```python
from build123d import *

# Parameters (mm, degrees)
SKETCH1_W            = 42
SKETCH1_H            = 33.02
BOSS_EXTRUDE1_DEPTH  = 0.381
SKETCH3_R            = 1.2192
CUT_EXTRUDE2_DEPTH   = 1.5875
CUT_EXTRUDE1_REACH   = 28.724
CUT_EXTRUDE3_START   = -0.762
CUT_EXTRUDE3_DEPTH   = 0.762
FILLET1_R            = 1.27
CUT_EXTRUDE4_REACH   = 28.724
SKETCH7_R            = 0.7874
FILLET1_OF_MIRROR1_R = 1.27
MIRROR2_START        = -0.381
MIRROR2_DEPTH        = 0.762
SKETCH6_W            = 2.5
SKETCH6_H            = 9.525
BOSS_EXTRUDE2_DEPTH  = 0.0254
CIRPATTERN1_COUNT    = 2


# Read off the part's stored shape, not the designer's step: Mirror2
with BuildPart() as part:
    # Sketch1 → Boss-Extrude1 (new, symmetric)
    with BuildSketch(Plane(origin=(0, 0, 0), x_dir=(1, 0, 0), z_dir=(0, 1, 0))):
        Rectangle(SKETCH1_W, SKETCH1_H)
    extrude(amount=BOSS_EXTRUDE1_DEPTH, both=True)

    # Sketch3 → Cut-Extrude2 (cut)
    with BuildSketch(Plane(origin=(0, 0.381, 0), x_dir=(1, 0, 0), z_dir=(0, 1, 0))):
        with Locations(Location((0, 0, 0), (0, 0, 270))):
            Circle(SKETCH3_R)
    extrude(amount=-CUT_EXTRUDE2_DEPTH, mode=Mode.SUBTRACT)

    # Sketch2 → Cut-Extrude1 (cut, up to next)
    with BuildSketch(Plane(origin=(0, 0.381, 0), x_dir=(1, 0, 0), z_dir=(0, 1, 0)), mode=Mode.PRIVATE) as cut_extrude1_sk1:
        with BuildLine():
            Line((9.144, 16.51), (9.144, 15.45082))
            ThreePointArc((9.144, 15.45082), (7.747, 14.05382), (6.35, 15.45082))
            Line((6.35, 15.45082), (6.35, 16.51))
            ThreePointArc((6.35, 16.51), (7.747, 17.907), (9.144, 16.51))
        make_face()
    cut_extrude1_tool1 = extrude(cut_extrude1_sk1.sketch, amount=-CUT_EXTRUDE1_REACH, mode=Mode.PRIVATE) & part.part
    cut_extrude1 = cut_extrude1_tool1.solids().sort_by_distance((7.747, 0.381, -15.98041))[0]
    add(cut_extrude1, mode=Mode.SUBTRACT)

    # Sketch5 → Cut-Extrude3 (cut)
    with BuildSketch(Plane(origin=(0, 0.381, 0), x_dir=(1, 0, 0), z_dir=(0, 1, 0)).offset(CUT_EXTRUDE3_START)):
        Polygon((21, 4.7625), (21, -4.7625), (14.24559, -4.7625), (14.24559, -19.569767896), (25.307623141, -19.569767896), (25.307623141, 18.786679146), (14.24559, 18.786679146), (14.24559, 4.7625), align=None)
    cut_extrude3 = extrude(amount=CUT_EXTRUDE3_DEPTH, mode=Mode.SUBTRACT)

    # Fillet1
    fillet1_edges = [part.edges().sort_by_distance(p)[0] for p in [
        (14.24559, 0, 4.7625),
        (14.24559, 0, -4.7625),
    ]]
    fillet(fillet1_edges, radius=FILLET1_R)

    # Sketch7 → Cut-Extrude4 (cut, up to next)
    with BuildSketch(Plane(origin=(0, 0.381, 0), x_dir=(1, 0, 0), z_dir=(0, 1, 0)), mode=Mode.PRIVATE) as cut_extrude4_sk1:
        with Locations(Location((4.826, 14.732, 0), (0, 0, 270))):
            Circle(SKETCH7_R)
    cut_extrude4_tool1 = extrude(cut_extrude4_sk1.sketch, amount=-CUT_EXTRUDE4_REACH, mode=Mode.PRIVATE) & part.part
    cut_extrude4 = cut_extrude4_tool1.solids().sort_by_distance((4.826, 0.381, -14.732))[0]
    add(cut_extrude4, mode=Mode.SUBTRACT)

    # Mirror1: Cut-Extrude1, Cut-Extrude3 across plane
    add(cut_extrude1.mirror(Plane(origin=(0, 0, 0), x_dir=(0, 0, 1), z_dir=(1, 0, 0))), mode=Mode.SUBTRACT)
    add(cut_extrude3.mirror(Plane(origin=(0, 0, 0), x_dir=(0, 0, 1), z_dir=(1, 0, 0))), mode=Mode.SUBTRACT)

    # Fillet1 of Mirror1
    fillet1_of_mirror1_edges = [part.edges().sort_by_distance(p)[0] for p in [
        (-14.24559, 0, 4.7625),
        (-14.24559, 0, -4.7625),
    ]]
    fillet(fillet1_of_mirror1_edges, radius=FILLET1_OF_MIRROR1_R)

    # Mirror2 outline → Mirror2 (cut)
    with BuildSketch(Plane(origin=(0, 0, 0), x_dir=(1, 0, 0), z_dir=(0, 1, 0)).offset(MIRROR2_START)):
        with BuildLine():
            Line((-9.144, -16.51), (-6.35, -16.51))
            Line((-6.35, -16.51), (-6.35, -15.45082))
            ThreePointArc((-6.35, -15.45082), (-7.747, -14.05382), (-9.144, -15.45082))
            Line((-9.144, -15.45082), (-9.144, -16.51))
        make_face()
        with BuildLine():
            Line((9.144, -16.51), (9.144, -15.45082))
            ThreePointArc((9.144, -15.45082), (7.747, -14.05382), (6.35, -15.45082))
            Line((6.35, -15.45082), (6.35, -16.51))
            Line((6.35, -16.51), (9.144, -16.51))
        make_face()
    extrude(amount=MIRROR2_DEPTH, mode=Mode.SUBTRACT)

    # Sketch6 → Boss-Extrude2 (add)
    with BuildSketch(Plane(origin=(0, -0.381, 0), x_dir=(1, 0, 0), z_dir=(0, 1, 0))):
        with Locations((-19.75, 0)):
            Rectangle(SKETCH6_W, SKETCH6_H)
        with Locations((-15.98, 0)):
            Rectangle(SKETCH6_W, SKETCH6_H)
    boss_extrude2 = extrude(amount=-BOSS_EXTRUDE2_DEPTH)

    # Mirror3: Boss-Extrude2 across plane
    add(boss_extrude2.mirror(Plane(origin=(0, 0, 0), x_dir=(0, 0, 1), z_dir=(1, 0, 0))))

    # CirPattern1: Cut-Extrude4 ×2 about axis
    cirpattern1_axis = Axis((0, 0, 0), (0, 1, 0))
    for i in range(1, CIRPATTERN1_COUNT):
        add(cut_extrude4.rotate(cirpattern1_axis, i * 360 / CIRPATTERN1_COUNT), mode=Mode.SUBTRACT)


solid = part.part
```
Can you work these out from the model? Positions are in its coordinate system, mm. Round coordinates to 2 decimals unless told otherwise and drop trailing zeros. Loops run counter-clockwise (first coordinate to the right, second up) from the corner with the lowest first, then second, coordinate; pieces in that order, holes last. Notation, with made-up numbers: M 31,36 L 57,36 A11 cw 57,40 Z; hole C 57.5,20 d2. An arc over 180 degrees is marked long. Answer in a Markdown table with one row per item.
1. If we section it at C-C, the plane z = -14.5: Please give me the cut outline in (x, y), plus the area to 3 significant figures.
Established:
| item | result |
|---|---|
| outline | M -14.25,-0.38 L -8.77,-0.38 L -8.77,0.38 L -14.25,0.38 Z; M -6.72,-0.38 L 4.07,-0.38 L 4.07,0.38 L -6.72,0.38 Z; M 5.58,-0.38 L 6.72,-0.38 L 6.72,0.38 L 5.58,0.38 Z; M 8.77,-0.38 L 14.25,-0.38 L 14.25,0.38 L 8.77,0.38 Z |
| area | 17.4 mm² |
2. I'm going to push a flat-ended pin straight in: pin 1 Ø2 at (x, z) = (4.826, -14.732) entering from -Y. Where does the tip first touch, or does it pass through?
Established:
| item | result |
|---|---|
| pin 1 | y = -0.38 |
3. Thinking about a two-plate mould opening in Z: for faces 1 (the face through (-4.524, 0.005, 14.005)), 2 (the face through (-20, -0.406, 0)), 3 (the face through (-7.716, -0.005, 14.054)), which applies, pulls with the +Z half, pulls with the -Z half, needs draft (parallel to the pull), parting line crosses it, or undercut?
Established:
| item | result |
|---|---|
| face 1 | undercut |
| face 2 | needs draft |
| face 3 | pulls with the +Z half |
4. Please list where these lines run through material, in increasing order: line 1 (X direction, y = 0.35, z = -13); line 2 (Y direction, x = 4, z = 11.5); line 3 (Z direction, x = -0.5, y = 0.05). Write a range as from..to.
Established:
| item | result |
|---|---|
| line 1 | -14.25..14.25 |
| line 2 | -0.38..0.38 |
| line 3 | -16.51..-1.11, 1.11..16.51 |
5. If we section it at D-D, the plane y = -0.2: Give the number of separate pieces and of enclosed holes in the cut face, plus the area to 3 significant figures.
Established:
| item | result |
|---|---|
| separate pieces | 1 |
| enclosed holes | 3 |
| area | 1,040 mm² |
6. If we section it at B-B, the plane x = 0: Please give me the cut outline in (y, z).
Established:
| item | result |
|---|---|
| outline | M -0.38,-16.51 L 0.38,-16.51 L 0.38,-1.22 L -0.38,-1.22 Z; M -0.38,1.22 L 0.38,1.22 L 0.38,16.51 L -0.38,16.51 Z |
